The listing builds one solid part. Answer for the finished solid, in the listing's coordinates (mm). A direction names the side the tool comes from. Round coordinates to 2 decimals unless told otherwise and drop trailing zeros. Write each loop counter-clockwise with the first axis right and the second up, starting at its lowest first coordinate (ties: lowest second). Pieces come first, ordered by that corner, then holes. Notation, with made-up numbers: (38, 17) - (97, 17) arc R13 ccw to (97, 35) - close; hole circle Ø11 at (14.25, 32). An arc over 180 degrees is marked (long way). Use a Markdown table: item, result. Add a question column.
1) A cutting plane is placed at C-C (x = 67). Give the vertices of the cut face in (y, z), then the cut area to 3 significant figures.
2) Each of these flat-tipped pins is pushed along its axis until it touches: P1, Ø14.5, axis at x = 57.5, y = 9.5, coming from the +Z side; P2, Ø6, axis at x = -6, z = 46, coming from the +Y side; P3, Ø10, axis at x = 13.5, z = 50.5, coming from the -Y side. Where does it stop, or does it pass through?
3) A cutting plane is placed at B-B (z = 2). Give the vertices of the cut face in (x, y), then the cut area to 3 significant figures.
4) A tool of negligible diameter and unlimited length cuts with its end or side. For faces 1 (the cylindrical face through (31.94, 16.55, 57.72)), 2 (the flat face through (44.45, -1, 8)), 3 (the flat face through (41, -25.4, 41)), 4 (the cylindrical face through (31.94, -16.79, 57.72)), from which of +Z, -Z, +X, -X, +Y, -Y can it reach the whole face along a straight path? Write none if from no direction.
5) A cutting plane is placed at A-A (y = 19). Give the vertices of the cut face in (x, z) (3 decimals), then the cut area to 3 significant figures.
6) Find the intervals of material crossed by probe 1 along Z at (x, y) = (64.5, 21); probe 2 along Z at (x, y) = (-13, 43) (3 decimals); probe 3 along X at (y, z) = (27.5, 2), in increasing order. Write a range as from..to.
```python
from build123d import *

# Parameters (mm, degrees)
F1_DEPTH = 63.5
F2_DEPTH = 25.4
F3_DEPTH = 7.9375
F0_W     = 23.8009692669
F0_H     = 19.05


with BuildPart() as f1:
    # F0 (on Front) → F1 (new body, symmetric)
    with BuildSketch(Plane.XZ):
        Polygon((25.4, 9.525), (-44.45, 9.525), (-44.45, -9.525), (44.45, -9.525), (44.45, 9.525), align=None)
    extrude(amount=F1_DEPTH, both=True)

    # F0 (on Front) → F2 (join, symmetric)
    with BuildSketch(Plane.XZ):
        with BuildLine():
            Line((25.4, 37.3717802988), (25.4, 9.525))
            Line((25.4, 9.525), (44.45, 9.525))
            Line((44.45, 9.525), (44.45, 37.3717802988))
            ThreePointArc((44.45, 37.3717802988), (49.0996798487, 48.5971004502), (60.325, 53.2467802988))
            Line((60.325, 53.2467802988), (65.0990307331, 53.2467802988))
            Line((65.0990307331, 53.2467802988), (65.0990307331, 72.2967802988))
            Line((65.0990307331, 72.2967802988), (60.325, 72.2967802988))
            ThreePointArc((60.325, 72.2967802988), (35.6292956671, 62.0674846318), (25.4, 37.3717802988))
        make_face()
    extrude(amount=F2_DEPTH, both=True)

    # F0 (on Front) → F3 (join, symmetric)
    with BuildSketch(Plane.XZ):
        with BuildLine():
            add(Edge.make_bspline(
                [(-44.45, 9.525), (-43.8166595995, 50.4934750497), (21.2823729962, 74.2796584964), (60.325, 72.2967802988)],
                knots=[0, 0, 0, 0, 122.139661973, 122.139661973, 122.139661973, 122.139661973], degree=3))
            Line((-44.45, 9.525), (25.4, 9.525))
            Line((25.4, 9.525), (25.4, 37.3717802988))
            ThreePointArc((25.4, 37.3717802988), (35.6292956671, 62.0674846318), (60.325, 72.2967802988))
        make_face()
    extrude(amount=F3_DEPTH, both=True)

    # F0 (on Front) → F4 (revolve)
    with BuildSketch(Plane.XZ):
        with Locations((76.9995153666, 62.7717802988)):
            Rectangle(F0_W, F0_H)
    revolve(axis=Axis((65.0990307331, 0, 63.4473668933), (0, 0, -1)))


solid = f1.part
```
Entries:
| question | item | result |
|---|---|---|
| 1 | outline | (-23.72, 53.25) - (23.72, 53.25) - (23.72, 72.3) - (-23.72, 72.3) - close |
| 1 | area | 904 mm² |
| 2 | P1 | stops at z = 72.41 |
| 2 | P2 | stops at y = 7.94 |
| 2 | P3 | stops at y = -7.94 |
| 3 | outline | (-44.45, -63.5) - (44.45, -63.5) - (44.45, 63.5) - (-44.45, 63.5) - close |
| 3 | area | 11,300 mm² |
| 4 | face 1 | +Z, -X, +Y |
| 4 | face 2 | -Z, +X, +Y, -Y |
| 4 | face 3 | +Z, +X, -X, -Y |
| 4 | face 4 | +Z, -X, -Y |
| 5 | outline | (-44.45, -9.525) - (44.45, -9.525) - (44.45, 37.372) arc R15.875 cw to (60.325, 53.247) - (79.434, 53.247) - (79.434, 72.297) - (50.764, 72.297) - (50.764, 70.963) arc R34.925 ccw to (25.4, 37.372) - (25.4, 9.525) - (-44.45, 9.525) - close |
| 5 | area | 3,350 mm² |
| 6 | probe 1 | z = 53.25..72.3 |
| 6 | probe 2 | z = -9.525..9.525 |
| 6 | probe 3 | x = -44.45..44.45 |
